Can you work these out from the model? Positions are in its coordinate system, mm. A direction names the side the tool comes from. Coordinates: 2 decimals unless noted, no trailing zeros. Order: outer loops, then holes, each group sorted by start corner. A loop starts at its lowest first (then second) coordinate and runs counter-clockwise, first axis right, second up. Notation, with made-up numbers: (47.5, 62) - (100.5, 62) arc R24 ccw to (100.5, 80) - close; hole circle Ø2 at (2.5, 70). An arc over 180 degrees is marked (long way). Use a Markdown table: item, result. Add a question column.
(1) I want a section at B-B (x = 77.5). List the corners of the cut face in (y, z) for me.
(2) I want a section at C-C (z = 29). List the corners of the cut face in (x, y) for me.
(3) If I drill on L1, parallel to Z at x = 80, y = -19.5; L2, parallel to X at y = -12.75, z = 76; L3, parallel to X at y = -24, z = 65.5, over which ranges is the centre line in solid material (lowest first)? Write a range as [from, to].
(4) I want a section at A-A (y = -14). List the corners of the cut face in (x, z) for me, and give its area (3 significant figures).
(5) For pin 1 Ø7.5 at (x, y) = (78.5, -16.5) entering from -Z; pin 2 Ø8 at (x, y) = (46.5, -18) entering from -Z; pin 3 Ø2.5 at (y, z) = (-8.5, 80.5) entering from -X, each with a flat end and sliding along its axis, tell me the tip position at first contact or that it passes through.
(6) On a 3-axis mill with a long thin cutter (end or side, diameter ignored), from which of +Z, -Z, +X, -X, +Y, -Y can I reach the whole of each face in a straight line? I mean faces 1 (the flat face through (37.166, -13, 29)), 2 (the flat face through (73, -13, 83.347)). Say none if no direction works.
```python
from build123d import *

# Parameters (mm, degrees)
F1_DEPTH = 25.4


with BuildPart() as f1:
    # F0 (on Front) → F1 (new body)
    with BuildSketch(Plane.XZ):
        Polygon((56.856412, 74.760954), (56.856412, 55.710954), (88.627096, 55.710954), (88.627096, 83.346918), (56.856412, 83.346918), align=None)
        with BuildLine():
            Line((-30.933438, 21.966385), (18.116245, 21.966385))
            Line((18.116245, 21.966385), (18.116245, 36.020787))
            ThreePointArc((18.116245, 36.020787), (29.462977, 63.414222), (56.856412, 74.760954))
            ThreePointArc((56.856412, 74.760954), (4.674775, 62.14329), (-30.933438, 21.966385))
        make_face()
        with BuildLine():
            Line((18.116245, 21.966385), (37.166245, 21.966385))
            Line((37.166245, 21.966385), (37.166245, 36.020787))
            ThreePointArc((37.166245, 36.020787), (42.933361, 49.943838), (56.856412, 55.710954))
            Line((56.856412, 55.710954), (56.856412, 74.760954))
            ThreePointArc((56.856412, 74.760954), (29.462977, 63.414222), (18.116245, 36.020787))
            Line((18.116245, 36.020787), (18.116245, 21.966385))
        make_face()
    extrude(amount=F1_DEPTH)


solid = f1.part
```
Answers follow:
| question | item | result |
|---|---|---|
| 1 | outline | (-25.4, 55.71) - (0, 55.71) - (0, 83.35) - (-25.4, 83.35) - close |
| 2 | outline | (-27.41, -25.4) - (37.17, -25.4) - (37.17, 0) - (-27.41, 0) - close |
| 3 | L1 | z = [55.71, 83.35] |
| 3 | L2 | x = [56.86, 88.63] |
| 3 | L3 | x = [10.78, 88.63] |
| 4 | outline | (-30.93, 21.97) - (37.17, 21.97) - (37.17, 36.02) arc R19.69 cw to (56.86, 55.71) - (88.63, 55.71) - (88.63, 83.35) - (56.86, 83.35) - (56.86, 74.76) arc R89.62 ccw to start |
| 4 | area | 3,730 mm² |
| 5 | pin 1 | stops at z = 55.71 |
| 5 | pin 2 | stops at z = 49.5 |
| 5 | pin 3 | stops at x = 56.86 |
| 6 | face 1 | -Z, +X, +Y, -Y |
| 6 | face 2 | +Z, +X, -X, +Y, -Y |
